from build123d import *

# Parameters (mm, degrees)
F1_DEPTH = 20
F3_D     = 10
F2_R     = 18
F4_DEPTH = 30
F6_D     = 16
F6_DEPTH = 25
F6_TIP   = 4.8068849522


with BuildPart() as f1:
    # F0 (on Top) → F1 (new body)
    with BuildSketch(Plane.XY):
        with BuildLine():
            Line((-10.7142857143, 22.5876975726), (-39.2857142857, 9.0350790291))
            ThreePointArc((-39.2857142857, 9.0350790291), (-45, 0), (-39.2857142857, -9.0350790291))
            Line((-39.2857142857, -9.0350790291), (-10.7142857143, -22.5876975726))
            ThreePointArc((-10.7142857143, -22.5876975726), (0, -25), (10.7142857143, -22.5876975726))
            Line((10.7142857143, -22.5876975726), (39.2857142857, -9.0350790291))
            ThreePointArc((39.2857142857, -9.0350790291), (45, 0), (39.2857142857, 9.0350790291))
            Line((39.2857142857, 9.0350790291), (10.7142857143, 22.5876975726))
            ThreePointArc((10.7142857143, 22.5876975726), (0, 25), (-10.7142857143, 22.5876975726))
        make_face()
    extrude(amount=F1_DEPTH)

    # F3 (through all)
    with Locations(Plane.XY.offset(20)):
        with Locations((-35, 0), (35, 0)):
            Hole(F3_D / 2)

    # F2 (on face) → F4 (join)
    with BuildSketch(Plane.XY.offset(20)):
        Circle(F2_R)
    extrude(amount=F4_DEPTH)

    # F6
    with Locations(Plane.XY.offset(50)):
        with Locations((0, 0)):
            Hole(F6_D / 2, depth=F6_DEPTH)
            with Locations((0, 0, -(F6_DEPTH + F6_TIP / 2))):  # 118° drill point
                Cone(0, F6_D / 2, F6_TIP, mode=Mode.SUBTRACT)


solid = f1.part
Part model, mm, in its own coordinate system. A direction names the side the tool comes from. Round coordinates to 2 decimals unless told otherwise and drop trailing zeros. Order: outer loops, then holes, each group sorted by start corner. A loop starts at its lowest first (then second) coordinate and runs counter-clockwise, first axis right, second up. Notation, with made-up numbers: (-9, 39.25) -> (49, 39.25) arc R27 cw to (49, 66.25) -> close; hole circle Ø8 at (79.25, 41.5). An arc over 180 degrees is marked (long way). Put each result on its own line as item: value.
Q1. Tool access for faces 1 (the face through (-11, 17, 20)), 2 (the face through (-25.2, -15.717, 9.86)): list every direction of +Z, -Z, +X, -X, +Y, -Y with a clear straight run to the whole face (end or side of a thin tool).
From the geometry:
face 1: +Z
face 2: +Z, -Z, -X, -Y
Q2. Band-saw the part on C-C (y = 10.5). Give the cut face in (x, z), and give its area (3 significant figures).
From the geometry:
outline: (-36.2, 0) -> (36.2, 0) -> (36.2, 20) -> (14.62, 20) -> (14.62, 50) -> (-14.62, 50) -> (-14.62, 20) -> (-36.2, 20) -> close
area: 2,330 mm2
Q3. Pull direction X, two halves, no side cores. Call faces 3 (the face through (-2.343, 17.847, 34.79)), 4 (the face through (25.2, 15.717, 9.86)), 5 (the face through (8, -4, 50)), 6 (the face through (1.73, -7.81, 37.33)): pulls with the +X half, pulls with the -X half, needs draft (parallel to the pull), parting line crosses it, or undercut.
From the geometry:
face 3: parting line crosses it
face 4: pulls with the +X half
face 5: needs draft
face 6: undercut
Q4. Band-saw the part on B-B (x = -35). Give the cut face in (y, z), and give its area (3 significant figures).
From the geometry:
outline: (-11.07, 0) -> (-5, 0) -> (-5, 20) -> (-11.07, 20) -> close; (5, 0) -> (11.07, 0) -> (11.07, 20) -> (5, 20) -> close
area: 243 mm2
Q5. Pin check, flat tips, straight feed: pin 1 Ø1 at (x, z) = (-22.5, 11) entering from +Y; pin 2 Ø1.5 at (y, z) = (-12.5, 19.5) entering from -X; pin 3 Ø12 at (y, z) = (-18, 15.5) entering from -X. Stop position of each tip, or through.
From the geometry:
pin 1: stops at y = 17.23
pin 2: stops at x = -33.56
pin 3: stops at x = -33.04
Q6. Band-saw the part on A-A (z = 9.5). Give the cut face in (x, y).
From the geometry:
outline: (-39.29, -9.04) -> (-10.71, -22.59) arc R25 ccw to (10.71, -22.59) -> (39.29, -9.04) arc R10 ccw to (39.29, 9.04) -> (10.71, 22.59) arc R25 ccw to (-10.71, 22.59) -> (-39.29, 9.04) arc R10 ccw to start; hole circle Ø10 at (-35, 0); hole circle Ø10 at (35, 0)
Q7. Wall check: line 1 (Y direction, x = -35, z = 7); line 2 (Y direction, x = 36, z = 13); line 3 (Z direction, x = -15, y = 19.5). Give the ranges that are in metal, low to high. Write a range as [from, to].
From the geometry:
line 1: y = [-11.07, -5], [5, 11.07]
line 2: y = [-10.59, -4.9], [4.9, 10.59]
line 3: z = [0, 20]
Q8. Band-saw the part on D-D (z = 33). Give the cut face in (x, y).
From the geometry:
outline: circle Ø36 at (0, 0); hole circle Ø16 at (0, 0)
